The model under review builds one solid part; all positions refer to its coordinate system, in mm. A direction names the side the tool comes from. Coordinates: 2 decimals unless noted, no trailing zeros. Order: outer loops, then holes, each group sorted by start corner. A loop starts at its lowest first (then second) coordinate and runs counter-clockwise, first axis right, second up.
Autodesk Inventor part; units mm, degrees
ref_plane "YZ Plane" through (0, 0, 0) normal (1, 0, 0) x (0, 1, 0)
ref_plane "XZ Plane" through (0, 0, 0) normal (0, 1, 0) x (-1, 0, 0)
ref_plane "XY Plane" through (0, 0, 0) normal (0, 0, 1) x (1, 0, 0)
sketch "Sketch1" plane through (0, 0, 0) normal (0, 1, 0) x (-1, 0, 0)
  line L0 (7.3913, 8.6413) -> (-12.6087, 8.6413)
  line L1 (-12.6087, 8.6413) -> (-12.6087, -11.3587)
  line L2 (-12.6087, -11.3587) -> (7.3913, -11.3587)
  line L3 (7.3913, -11.3587) -> (7.3913, 8.6413)
  line L4 (5.3913, 6.6413) -> (-10.6087, 6.6413)
  line L5 (-10.6087, 6.6413) -> (-10.6087, -9.3587)
  line L6 (-10.6087, -9.3587) -> (5.3913, -9.3587)
  line L7 (5.3913, -9.3587) -> (5.3913, 6.6413)
  point P0 (0, 0)
  dimension "d0" = 20
  dimension "d1" = 20
  dimension "d2" = 2
  dimension "d3" = 2
  dimension "d4" = 2
  dimension "d5" = 2
extrude "Extrusion1" add sketch "Sketch1" along normal blind 300
sketch "Sketch2" plane through (-7.3913, 0, 8.6413) normal (0, 0, 1) x (1, 0, 0)
  circle A0 centre (10, 8) radius 1.5
  line L0 (0, 0) -> (0, 300)
  line L1 (0, 0) -> (20, 0)
  circle A1 centre (10, 260) radius 1.5
  line L2 (0, 300) -> (20, 300)
  point P0 (7.3913, 0)
  dimension "d8" = 3
  dimension "d9" = 10
  dimension "d10" = 8
  dimension "d28" = 3
  dimension "d29" = 10
  dimension "d30" = 40
hole "Hole1" at (2.6087, 8, 8.6413) at (2.6087, 260, 8.6413) direction (0, 0, -1) diameter 3 end through all
sketch "Sketch3" plane through (-7.3913, 0, -11.3587) normal (-1, 0, 0) x (0, 0, 1)
  circle A0 centre (10, 18.5) radius 1.5
  line L0 (0, 0) -> (20, 0)
  line L1 (0, 0) -> (0, 300)
  point P0 (11.3587, 0)
  dimension "d18" = 18.5
  dimension "d19" = 10
  dimension "d20" = 3
hole "Hole2" at (-7.3913, 18.5, -1.3587) direction (1, 0, 0) diameter 3 end through all
properties part number "profile_alu"
(1) Consider section B-B (y = 128). Give the boundary of the cut face in (x, z), then the cut area to 3 significant figures.
(2) Wall thickness on line 1 (X direction, y = 30.5, z = -1); line 2 (Z direction, x = -5.25, y = 31.5); line 3 (X direction, y = 260, z = -10.45): over which ranges is each line inside the solid? List them lowest first.
(3) Tool access review of faces 1 (the face through (-5.391, 148, -1)), 2 (the face through (-6, 300, -1)): name each direction out of +Z, -Z, +X, -X, +Y, -Y from which nothing blocks a thin tool from reaching the whole face with its end or side.
(4) Consider section A-A (x = 7.5). Give the boundary of the cut face in (y, z).
Findings:
1. outline: (-7.39, -11.36) - (12.61, -11.36) - (12.61, 8.64) - (-7.39, 8.64) - close; hole (-5.39, -9.36) - (10.61, -9.36) - (10.61, 6.64) - (-5.39, 6.64) - close
1. area: 144 mm2
2. line 1: x = -7.39 to -5.39, 10.61 to 12.61
2. line 2: z = -11.36 to -9.36, 6.64 to 8.64
2. line 3: x = -7.39 to 1.11, 4.11 to 12.61
3. face 1: +Y, -Y
3. face 2: +Z, -Z, +X, -X, +Y
4. outline: (0, -11.36) - (300, -11.36) - (300, -9.36) - (0, -9.36) - close; (0, 6.64) - (300, 6.64) - (300, 8.64) - (0, 8.64) - close
